The model under review builds one solid part; all positions refer to its coordinate system, in mm. Face numbers are marked on the shaded views. A direction names the side the tool comes from. Give positions to 0.01 mm unless a question says otherwise; leave off trailing zeros. Loops run counter-clockwise (first coordinate to the right, second up) from the corner with the lowest first, then second, coordinate; pieces in that order, holes last. Notation, with made-up numbers: M 16,28 L 68,28 A12 cw 68,48 Z; hole C -18,50.25 d11. An arc over 180 degrees is marked long. Write item = value, one per line. Start each with the question number.
1. We need section B-B on x = 10. Give the boundary of the cut face in (y, z), then the cut area to 3 significant figures.
2. For the marked faces 1, 2 and 3, list the 3-axis set-ups (+Z, -Z, +X, -X, +Y, -Y) from which the entire face can be reached by the end or side of a thin tool; tool diameter is ignored.
3. Wall thickness on line 1 along Y through (x, z) = (-31, 0.5); line 2 along X through (y, z) = (0.5, -5); line 3 along Y through (x, z) = (-37, 4.5): over which ranges is each line inside the solid? List them lowest first. Write a range as from..to.
4. We need section C-C on x = -50. Give the boundary of the cut face in (y, z).
5. For pin 1 (6 mm diameter, centred on x = -5, y = 2.5, fed in from -Z); pin 2 (4.5 mm diameter, centred on x = 1.5, z = -2.5, fed in from -Y); pin 3 (12 mm diameter, centred on x = -24.5, y = -1.5, fed in from +Z); pin 4 (2 mm diameter, centred on y = -0.5, z = -6.5, fed in from +X), all flat-tipped, find the tip position at first contact; note any pin that passes through.
6. We need section A-A on y = 0. Give the boundary of the cut face in (x, z), then the cut area to 3 significant figures.
from build123d import *

# Parameters (mm, degrees)
SKETCH_1_W          = 40
SKETCH_1_H          = 20
EXTRUDE_1_DEPTH     = 6
SKETCH_2_R          = 2.5
CUT_EXTRUDE_1_DEPTH = 24.151673806
EXTRUDE_START       = -15
EXTRUDE_2_OUTLINE_R = 11
EXTRUDE_2_DEPTH     = 15
EXTRUDE_START_2     = -8
SKETCH_5_R          = 11
SKETCH_5_R_2        = 10
EXTRUDE_3_DEPTH     = 8
SKETCH_8_W          = 15
SKETCH_8_H          = 5
EXTRUDE_4_DEPTH     = 200
SKETCH_9_W          = 4.403653586
SKETCH_9_H          = 3.736433346
EXTRUDE_5_DEPTH     = 15
SKETCH_13_W         = 87.445921981
SKETCH_13_H         = 18.524474632
CUT_EXTRUDE_2_DEPTH = 184.131783151
SKETCH_14_R         = 2.5
CUT_EXTRUDE_3_DEPTH = 10


# Read off the part's stored shape, not the designer's step: 凸台-拉伸2
with BuildPart() as part:
    # 草图1 → 凸台-拉伸1 (new body)
    with BuildSketch(Plane.XY):
        Rectangle(SKETCH_1_W, SKETCH_1_H)
    extrude(amount=EXTRUDE_1_DEPTH)

    # 草图2 → 切除-拉伸1 (cut, through all)
    with BuildSketch(Plane.XY.offset(6)):
        with Locations((10, 0)):
            Circle(SKETCH_2_R)
        with Locations((-1, 0)):
            Circle(SKETCH_2_R)
        with Locations((-12, 0)):
            Circle(SKETCH_2_R)
    extrude(amount=-CUT_EXTRUDE_1_DEPTH, mode=Mode.SUBTRACT)

    # 凸台-拉伸2 outline → 凸台-拉伸2 (add)
    with BuildSketch(Plane.XY.offset(6).offset(EXTRUDE_START)):
        with BuildLine():
            Line((20, 10), (20, 13.5))
            Line((20, 13.5), (-26.893967141, 13.5))
            Line((-26.893967141, 13.5), (-26.893967141, 13.384337644))
            ThreePointArc((-26.893967141, 13.384337644), (-45, 0), (-26.893967141, -13.384337644))
            Line((-26.893967141, -13.384337644), (-26.893967141, -13.5))
            Line((-26.893967141, -13.5), (20, -13.5))
            Line((20, -13.5), (20, -10))
            Line((20, -10), (-20, -10))
            Line((-20, -10), (-20, -8.660254038))
            ThreePointArc((-20, -8.660254038), (-17, 0), (-20, 8.660254038))
            Line((-20, 8.660254038), (-20, 10))
            Line((-20, 10), (20, 10))
        make_face()
        with Locations((-31, 0)):
            Circle(EXTRUDE_2_OUTLINE_R, mode=Mode.SUBTRACT)
    extrude(amount=EXTRUDE_2_DEPTH)

    # 草图5 → 凸台-拉伸3 (add)
    with BuildSketch(Plane.XY.offset(6).offset(EXTRUDE_START_2)):
        with Locations((-31, 0)):
            Circle(SKETCH_5_R)
        with Locations((-31, 0)):
            Circle(SKETCH_5_R_2, mode=Mode.SUBTRACT)
    extrude(amount=EXTRUDE_3_DEPTH)

    # 草图8 → 凸台-拉伸4 (add)
    with BuildSketch(Plane(origin=(20, 0, 0), x_dir=(0, 0, -1), z_dir=(1, 0, 0))):
        with Locations((1.5, 16)):
            Rectangle(SKETCH_8_W, SKETCH_8_H)
    extrude(amount=-EXTRUDE_4_DEPTH)

    # 草图9 → 凸台-拉伸5 (add, through all)
    with BuildSketch(Plane.XY.offset(6)):
        with Locations((-27.364497847, 13.796597935)):
            Rectangle(SKETCH_9_W, SKETCH_9_H)
    extrude(amount=-EXTRUDE_5_DEPTH)

    # 草图13 → 切除-拉伸2 (cut, through all)
    with BuildSketch(Plane(origin=(0, 18.5, 0), x_dir=(1, 0, 0), z_dir=(0, 1, 0))):
        with Locations((-139.388148112, 3.262237316)):
            Rectangle(SKETCH_13_W, SKETCH_13_H)
    extrude(amount=-CUT_EXTRUDE_2_DEPTH, mode=Mode.SUBTRACT)

    # 草图14 → 切除-拉伸3 (cut)
    with BuildSketch(Plane(origin=(0, 18.5, 0), x_dir=(1, 0, 0), z_dir=(0, 1, 0))):
        with Locations(Location((-85.665187121, 1.5, 0), (0, 0, 270))):
            Circle(SKETCH_14_R)
    extrude(amount=-CUT_EXTRUDE_3_DEPTH, mode=Mode.SUBTRACT)


solid = part.part
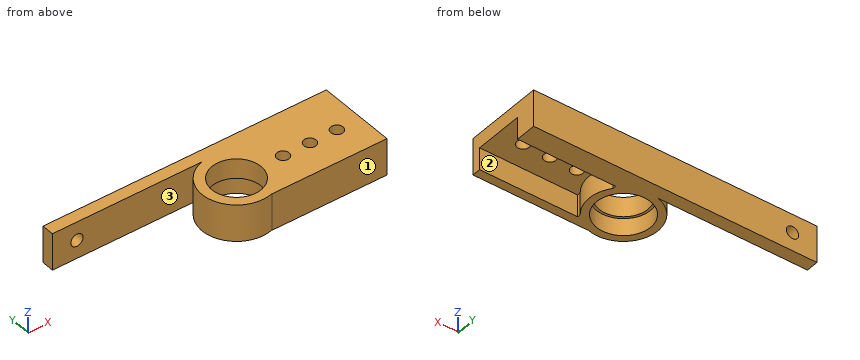
Final values:
q1.outline = M -13.5,-9 L -10,-9 L -10,0 L -2.5,0 L -2.5,6 L -13.5,6 Z; M 2.5,0 L 10,0 L 10,-9 L 18.5,-9 L 18.5,6 L 2.5,6 Z
q1.area = 270 mm²
q2.face_1 = +Z, -Z, +X, -Y
q2.face_2 = -Z, +X
q2.face_3 = +Z, -Z, -X
q3.line_1 = -14..-10, 10..18.5
q3.line_2 = -44.99..-41.99, -20.01..-17.01
q3.line_3 = -12.65..-8, 8..12.65, 13.5..18.5
q4.outline = M 13.5,-9 L 18.5,-9 L 18.5,6 L 13.5,6 Z
q5.pin_1 = 0
q5.pin_2 = -13.5
q5.pin_3 = 6
q5.pin_4 = -17
q6.outline = M -45,-9 L -42,-9 L -42,-2 L -41,-2 L -41,6 L -45,6 Z; M -21,-2 L -20,-2 L -20,-9 L -17,-9 L -17,0 L -14.5,0 L -14.5,6 L -21,6 Z; M -9.5,0 L -3.5,0 L -3.5,6 L -9.5,6 Z; M 1.5,0 L 7.5,0 L 7.5,6 L 1.5,6 Z; M 12.5,0 L 20,0 L 20,6 L 12.5,6 Z
q6.area = 238 mm²
